The model under review builds one solid part; all positions refer to its coordinate system, in mm. A direction names the side the tool comes from. Coordinates: 2 decimals unless noted, no trailing zeros. Write each loop counter-clockwise with the first axis right and the second up, starting at its lowest first coordinate (ties: lowest second). Pieces come first, ordered by that corner, then holes. Notation, with made-up numbers: (49, 40) -> (83, 40) arc R29 cw to (83, 72) -> close; hole circle Ø4 at (-35, 64). An arc over 180 degrees is marked (long way). Write each question's results on one line, items separated by ' | '.
```python
from build123d import *

# Parameters (mm, degrees)
F0_R     = 4.9022
F1_DEPTH = 133.35
F2_R     = 9.525
F3_DEPTH = 25.4
F4_R     = 12.7
F5_DEPTH = 12.7


with BuildPart() as f1:
    # F0 (on Front) → F1 (new body)
    with BuildSketch(Plane.XZ):
        Circle(F0_R)
    extrude(amount=-F1_DEPTH)

    # F2 (on Front) → F3 (join)
    with BuildSketch(Plane.XZ):
        Circle(F2_R)
    extrude(amount=F3_DEPTH)

    # F4 (on face) → F5 (join)
    with BuildSketch(Plane.XZ.offset(25.4)):
        Circle(F4_R)
    extrude(amount=F5_DEPTH)


solid = f1.part
```
Q1. Add section B-B (x = 0). Write out the cut boundary in (y, z) (3 decimals).
Solution:
outline: (-38.1, -12.7) -> (-25.4, -12.7) -> (-25.4, -9.525) -> (0, -9.525) -> (0, -4.902) -> (133.35, -4.902) -> (133.35, 4.902) -> (0, 4.902) -> (0, 9.525) -> (-25.4, 9.525) -> (-25.4, 12.7) -> (-38.1, 12.7) -> close
Q2. Clearance check with flat-ended pins moving along their axes: P1, Ø5, axis at y = 97.5, z = -2, coming from the +X side; P2, Ø4, axis at x = -2.5, y = 103, coming from the +Z side; P3, Ø1.5, axis at x = -1.5, y = 64.5, coming from the -Z side. State where each tip first meets the part, or that it passes through.
Solution:
P1: x = 4.9 | P2: z = 4.88 | P3: z = -4.84
Q3. Add section A-A (z = 0). Write out the cut boundary in (x, y) (3 decimals), plus the area to 3 significant figures.
Solution:
outline: (-12.7, -38.1) -> (12.7, -38.1) -> (12.7, -25.4) -> (9.525, -25.4) -> (9.525, 0) -> (4.902, 0) -> (4.902, 133.35) -> (-4.902, 133.35) -> (-4.902, 0) -> (-9.525, 0) -> (-9.525, -25.4) -> (-12.7, -25.4) -> close | area: 2,110 mm²
Q4. Machinability: for faces 1 (the flat face through (0, 133.35, 0)), 2 (the flat face through (4, 0, -4)), which of the approach directions +Z, -Z, +X, -X, +Y, -Y give a long, thin tool a straight path to every point of the face, cutting with its end or side? Answer none if there is none.
Solution:
face 1: +Z, -Z, +X, -X, +Y | face 2: +Y
Q5. Add section C-C (y = 119). Write out the cut boundary in (x, z), plus the area to 3 significant figures.
Solution:
outline: circle Ø9.8 at (0, 0) | area: 75.5 mm²
Q6. For line 1 (Y direction, x = 4.5, z = 2.5); line 2 (Y direction, x = 5.25, z = -11); line 3 (X direction, y = -4.5, z = 0.5), list the stretches that pass through material, from the lowest coordinate up. Write a range as from..to.
Solution:
line 1: -38.1..0 | line 2: -38.1..-25.4 | line 3: -9.51..9.51
